Job drawing, mm, ordinate dimensions from the low corner. One solid piece. A direction names the side the tool comes from. Coordinates: 2 decimals unless noted, no trailing zeros. Loops run counter-clockwise (first coordinate to the right, second up) from the corner with the lowest first, then second, coordinate; pieces in that order, holes last. Notation, with made-up numbers: (6.25, 10.5) - (36.25, 10.5) arc R28 ccw to (36.25, 29.5) - close; hole circle Ø1 at (-25, 38.5). An arc over 180 degrees is marked (long way). Use a Markdown table: item, result. Add a question column.
1) Drop flat-ended pins along their axis: P1, Ø1.4, axis at x = 27, y = 19.75, coming from the -Z side; P2, Ø0.9, axis at y = 1.5, z = 1, coming from the +X side; P3, Ø0.9, axis at x = 6.5, z = 1.5, coming from the -Y side. Give the stop position or say it passes through.
2) Pull direction X, two halves, no side cores. Call the marked faces 4 and 5: +X half, -X half, draft (parallel to the pull), parting line (faces both ways), or undercut.
3) Tool access for the marked faces 1, 2 and 3: list every direction of +Z, -Z, +X, -X, +Y, -Y with a clear straight run to the whole face (end or side of a thin tool).
4) Band-saw the part on B-B (y = 8.5). Give the cut face in (x, z).
5) Probe probe 1 along Y at (x, z) = (20.5, 2.45); probe 2 along X at (y, z) = (2.5, 1.95); probe 3 along X at (y, z) = (19.25, 1) (1 decimal). List the from-to ranges inside material, lowest first. Write a range as [from, to].
6) Band-saw the part on D-D (x = 20.75). Give the cut face in (y, z).
7) Band-saw the part on C-C (z = 1.95). Give the number of separate pieces and of enclosed holes in the cut face, plus the area to 3 significant figures.
8) Band-saw the part on A-A (y = 12.25). Give the cut face in (x, z) (1 decimal), plus the area to 3 significant figures.
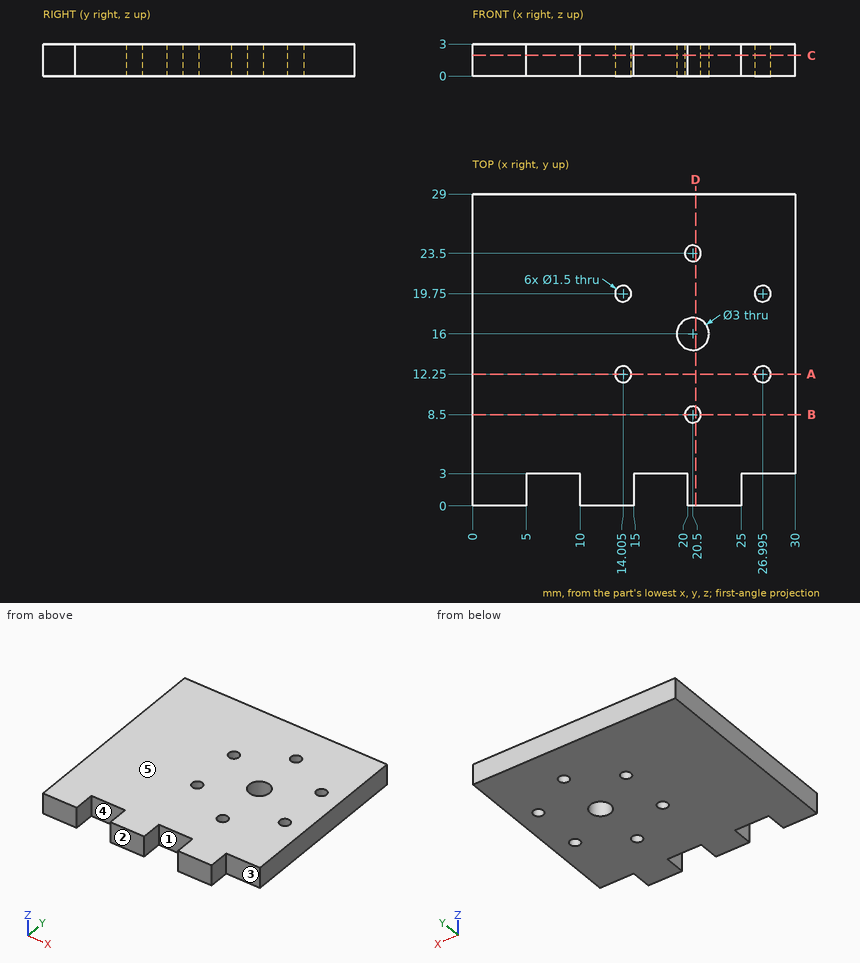
Answer block:
| question | item | result |
|---|---|---|
| 1 | P1 | through |
| 1 | P2 | x = 25 |
| 1 | P3 | y = 3 |
| 2 | face 4 | undercut |
| 2 | face 5 | draft |
| 3 | face 1 | +Z, -Z, -Y |
| 3 | face 2 | +Z, -Z, +X, -X, -Y |
| 3 | face 3 | +Z, -Z, +X, -Y |
| 4 | outline | (0, 0) - (19.75, 0) - (19.75, 3) - (0, 3) - close; (21.25, 0) - (30, 0) - (30, 3) - (21.25, 3) - close |
| 5 | probe 1 | [0, 7.75], [9.25, 14.5], [17.5, 22.75], [24.25, 29] |
| 5 | probe 2 | [0, 5], [10, 15], [20, 25] |
| 5 | probe 3 | [0, 13.4], [14.6, 26.4], [27.6, 30] |
| 6 | outline | (0, 0) - (7.79, 0) - (7.79, 3) - (0, 3) - close; (9.21, 0) - (14.52, 0) - (14.52, 3) - (9.21, 3) - close; (17.48, 0) - (22.79, 0) - (22.79, 3) - (17.48, 3) - close; (24.21, 0) - (29, 0) - (29, 3) - (24.21, 3) - close |
| 7 | separate pieces | 1 |
| 7 | enclosed holes | 7 |
| 7 | area | 807 mm2 |
| 8 | outline | (0, 0) - (13.3, 0) - (13.3, 3) - (0, 3) - close; (14.8, 0) - (26.2, 0) - (26.2, 3) - (14.8, 3) - close; (27.7, 0) - (30, 0) - (30, 3) - (27.7, 3) - close |
| 8 | area | 81.0 mm2 |
